Read the model definition and answer for the solid it produces. Units are mm, in the model's axes. A direction names the side the tool comes from. Coordinates: 2 decimals unless noted, no trailing zeros. Loops run counter-clockwise (first coordinate to the right, second up) from the corner with the lowest first, then second, coordinate; pieces in that order, holes last. Notation, with made-up numbers: (-8, -35.75) - (28, -35.75) arc R23 cw to (28, -9.75) - close; hole circle Ø6 at (88, -15). An arc over 180 degrees is marked (long way). Use one line per item in the form item = value.
Autodesk Inventor part; units mm, degrees
ref_plane "YZ Plane" through (0, 0, 0) normal (1, 0, 0) x (0, 1, 0)
ref_plane "XZ Plane" through (0, 0, 0) normal (0, 1, 0) x (-1, 0, 0)
ref_plane "XY Plane" through (0, 0, 0) normal (0, 0, 1) x (1, 0, 0)
sketch "Sketch1" plane through (0, 0, 0) normal (0, 1, 0) x (-1, 0, 0)
  line L0 (0, 0) -> (8, 0)
  line L1 (8, -10) -> (0, -10)
  line L2 (0, -10) -> (0, 0)
  line L3 (8, -1) -> (1, -1)
  line L4 (1, -1) -> (1, -9)
  line L5 (1, -9) -> (8, -9)
  line L6 (8, 0) -> (8, -1)
  line L7 (8, -9) -> (8, -10)
  dimension "d0" = 1
  dimension "d1" = 1
  dimension "d2" = 1
  dimension "d3" = 10
  dimension "d4" = 8
extrude "Extrusion1" add sketch "Sketch1" along normal blind 410
sketch "Sketch2" plane through (0, 0, 0) normal (1, 0, 0) x (0, 0, -1)
  line L0 (0, 0) -> (10, 0)
  line L1 (0, 0) -> (0, 410)
  point P0 (5, 10)
  dimension "d7" = 10
  dimension "d8" = 5
hole "Hole1" at (0, 10, -5) direction (-1, 0, 0) diameter 3 depth 8 tip angle 118
sketch "Sketch3" plane through (0, 0, 0) normal (1, 0, 0) x (0, 0, -1)
  line L0 (0, 0) -> (0, 410)
  line L1 (0, 410) -> (10, 410)
  point P0 (5, 277.5)
  point P1 (5, 410)
  dimension "d16" = 5
  dimension "d17" = 132.5
hole "Hole2" at (0, 277.5, -5) direction (-1, 0, 0) diameter 3 depth 8 tip angle 118
sketch "Sketch5" plane through (0, 0, 0) normal (1, 0, 0) x (0, 0, -1)
  line L0 (0, 0) -> (0, 410)
  circle A0 centre (5, 10) radius 1.5
  point P0 (5, 200)
  dimension "d25" = 5
  dimension "d26" = 190
hole "Hole3" at (0, 200, -5) direction (-1, 0, 0) diameter 3 depth 8 tip angle 118
properties part number "Stringer" material "Aluminum"
Item 1: Each of these flat-tipped pins is pushed along its axis until it touches: P1, Ø4, axis at y = 10, z = -5, coming from the -X side; P2, Ø2.5, axis at y = 277.5, z = -5, coming from the +X side. Where does it stop, or does it pass through?
Results below:
P1 = -1
P2 = through
Item 2: The part is cut by section B-B on x = -2.5. Give the vertices of the cut face in (y, z).
Results below:
outline = (0, -10) - (410, -10) - (410, -9) - (0, -9) - close; (0, -1) - (410, -1) - (410, 0) - (0, 0) - close
Item 3: Which of the six approach directions +Z, -Z, +X, -X, +Y, -Y give full straight-line access (tool end or side, diameter ignored) to faces 1 (the flat face through (-0.7, 410, -5)), 2 (the flat face through (-4, 202, -9))?
Results below:
face_1 = +Z, -Z, +X, -X, +Y
face_2 = -X, +Y, -Y
Item 4: For a pull along Z with two mould halves and no side action, classify faces 3 (the flat face through (-0.7, 0, -5)), 4 (the flat face through (-4, 202, -10)), 5 (the flat face through (-5, 202, -1)) as +Z half, -Z half, draft (parallel to the pull), parting line (faces both ways), or undercut.
Results below:
face_3 = draft
face_4 = -Z half
face_5 = undercut
Item 5: The part is cut by section C-C on y = 167. Give the vertices of the cut face in (x, z), plus the area to 3 significant figures.
Results below:
outline = (-8, -10) - (0, -10) - (0, 0) - (-8, 0) - (-8, -1) - (-1, -1) - (-1, -9) - (-8, -9) - close
area = 24.0 mm²
Item 6: Find the intervals of material crossed by L1, parallel to Y at x = -0.3, z = -5; L2, parallel to Z at x = -0.45, y = 200; L3, parallel to Z at x = -4.5, y = 338.5, in increasing order.
Results below:
L1 = 0 to 8.5, 11.5 to 198.5, 201.5 to 276, 279 to 410
L2 = -10 to -6.5, -3.5 to 0
L3 = -10 to -9, -1 to 0
Item 7: The part is cut by section A-A on z = -5. Give the vertices of the cut face in (x, y).
Results below:
outline = (-1, 0) - (0, 0) - (0, 8.5) - (-1, 8.5) - close; (-1, 11.5) - (0, 11.5) - (0, 198.5) - (-1, 198.5) - close; (-1, 201.5) - (0, 201.5) - (0, 276) - (-1, 276) - close; (-1, 279) - (0, 279) - (0, 410) - (-1, 410) - close
